```python
from build123d import *

# Parameters (mm, degrees)
F0_R     = 34.0995
F0_R_2   = 29.337
F1_DEPTH = 31.75
F0_R_3   = 25.527
F2_DEPTH = 7.9375
F3_R     = 30.1625
F3_R_2   = 25.4
F4_DEPTH = 6.35
F5_SIZE  = 2.54


with BuildPart() as f1:
    # F0 (on Top) → F1 (new body)
    with BuildSketch(Plane.XY):
        Circle(F0_R)
        Circle(F0_R_2, mode=Mode.SUBTRACT)
    extrude(amount=F1_DEPTH)

    # F0 (on Top) → F2 (join)
    with BuildSketch(Plane.XY):
        Circle(F0_R)
        Circle(F0_R_2, mode=Mode.SUBTRACT)
        Circle(F0_R_2)
        Circle(F0_R_3, mode=Mode.SUBTRACT)
    extrude(amount=-F2_DEPTH)

    # F3 (on face) → F4 (join)
    with BuildSketch(Plane(origin=(0, 0, -7.9375), x_dir=(1, 0, 0), z_dir=(0, 0, -1))):
        Circle(F3_R)
        Circle(F3_R_2, mode=Mode.SUBTRACT)
    extrude(amount=F4_DEPTH)

    # F5
    f5_edges = [f1.edges().sort_by_distance(p)[0] for p in [
        (-34.0995, 0, 31.75),
        (-34.0995, 0, -7.9375),
        (-30.1625, 0, -14.2875),
    ]]
    chamfer(f5_edges, length=F5_SIZE)


solid = f1.part
```
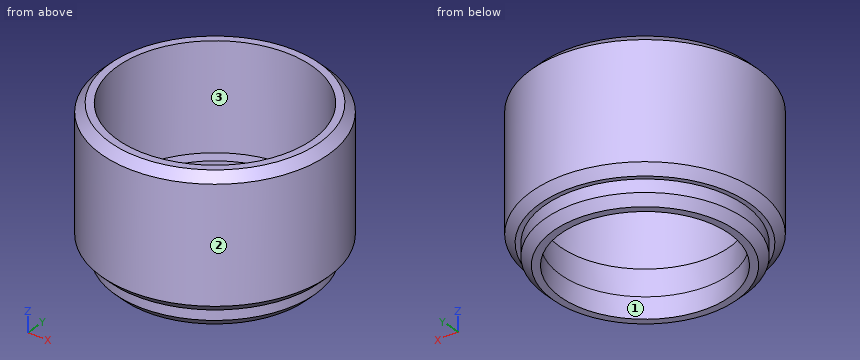
Geometry check sheet. Reference: the model listing, model coordinates, mm. Face numbers are marked on the shaded views. Coordinates: 2 decimals unless noted, no trailing zeros. Write each loop counter-clockwise with the first axis right and the second up, starting at its lowest first coordinate (ties: lowest second). Pieces come first, ordered by that corner, then holes. Notation, with made-up numbers: (88, -33) -> (145, -33) arc R21 ccw to (145, -5) -> close; hole circle Ø8 at (67, 76.25). An arc over 180 degrees is marked (long way). Use CSV: the item, a comma, the result in double quotes. Start each with the question number.
Item 1: Cross-section at C-C, the plane z = 7. Record the cut outline in (x, y), plus the area to 3 significant figures.
Item 2: Depth check by flat-ended pin: pin 1 Ø3 at (x, z) = (-8, 16.5) entering from +Y; pin 2 Ø1 at (y, z) = (11.5, 9.5) entering from -X; pin 3 Ø1.5 at (x, z) = (-19.5, 19) entering from -Y; pin 4 Ø15.5 at (x, y) = (12, -4) entering from +Z. Enter the tip coordinate at first touch or a pass-through.
Item 3: Thickness scan on line 1 (Y direction, x = 0, z = 21.5); line 2 (Y direction, x = 0, z = -11.5); line 3 (Z direction, x = -13.5, y = -23). Record the ranges inside material, lowest first.
Item 4: Mould release check, pull along Y, two halves, no side actions. Record for the marked faces 1, 2 and 3: released by +Y, released by -Y, zero draft, split by the parting line, or undercut.
Item 5: Cross-section at A-A, the plane x = 0. Record the cut outline in (y, z), plus the area to 3 significant figures.
Answers:
1,outline,"circle Ø68.2 at (0, 0); hole circle Ø58.67 at (0, 0)"
1,area,"949 mm^2"
2,pin 1,"y = 33.47"
2,pin 2,"x = -32.28"
2,pin 3,"y = -28.48"
2,pin 4,"through"
3,line 1,"-34.1 to -29.34, 29.34 to 34.1"
3,line 2,"-30.16 to -25.4, 25.4 to 30.16"
3,line 3,"-14.29 to 0"
4,face 1,"undercut"
4,face 2,"split by the parting line"
4,face 3,"undercut"
5,outline,"(-34.1, -5.4) -> (-31.56, -7.94) -> (-30.16, -7.94) -> (-30.16, -11.75) -> (-27.62, -14.29) -> (-25.4, -14.29) -> (-25.4, -7.94) -> (-25.53, -7.94) -> (-25.53, 0) -> (-29.34, 0) -> (-29.34, 31.75) -> (-31.56, 31.75) -> (-34.1, 29.21) -> close; (25.4, -14.29) -> (27.62, -14.29) -> (30.16, -11.75) -> (30.16, -7.94) -> (31.56, -7.94) -> (34.1, -5.4) -> (34.1, 29.21) -> (31.56, 31.75) -> (29.34, 31.75) -> (29.34, 0) -> (25.53, 0) -> (25.53, -7.94) -> (25.4, -7.94) -> close"
5,area,"480 mm^2"
